The listing builds one solid part. Answer for the finished solid, in the listing's coordinates (mm). Face numbers are marked on the shaded views. A direction names the side the tool comes from. Coordinates: 2 decimals unless noted, no trailing zeros. Order: outer loops, then holes, each group sorted by start corner. A loop starts at its lowest first (then second) coordinate and runs counter-clockwise, first axis right, second up. Notation, with made-up numbers: (66, 42) -> (113, 42) arc R16 ccw to (113, 48) -> close; hole circle Ø4 at (-20, 89). An arc over 180 degrees is marked (long way). Answer in a Markdown table with one row per item.
```python
from build123d import *

# Parameters (mm, degrees)
SKETCH_2_R          = 1.25
CUT_EXTRUDE_1_DEPTH = 10
CUT_EXTRUDE_START   = -54.1
SKETCH_2_2_R        = 1.25
CUT_EXTRUDE_2_DEPTH = 6
SKETCH_3_OUTSIDE_W  = 33.054
SKETCH_3_OUTSIDE_H  = 33.054
SKETCH_3_OUTSIDE_R  = 8.75
CUT_EXTRUDE_3_DEPTH = 20.1
SKETCH_4_R          = 5.25
SKETCH_4_R_2        = 4.25
EXTRUDE_1_DEPTH     = 4


with BuildPart() as part:
    # 草图1 → 旋转1 (revolve)
    with BuildSketch(Plane.XY, mode=Mode.PRIVATE) as revolve_1_sk:
        Polygon((-9, 36), (-5.25, 36), (-5.25, 5), (-9, 5), (-9, 0), (-4.25, 0), (-4.25, 60.1), (-9, 60.1), align=None)
    revolve(revolve_1_sk.sketch.rotate(Axis((0, 0, 0), (0, 1, 0)), 270), axis=Axis((0, 0, 0), (0, 1, 0)))

    # 草图2 → 切除-拉伸1 (cut)
    with BuildSketch(Plane(origin=(0, 60.1, 0), x_dir=(1, 0, 0), z_dir=(0, 1, 0))):
        with Locations(Location((0, 7, 0), (0, 0, 270))):
            Circle(SKETCH_2_R)
        with Locations(Location((0, -7, 0), (0, 0, 270))):
            Circle(SKETCH_2_R)
        with Locations(Location((-7, 0, 0), (0, 0, 270))):
            Circle(SKETCH_2_R)
        with Locations(Location((7, 0, 0), (0, 0, 270))):
            Circle(SKETCH_2_R)
    extrude(amount=-CUT_EXTRUDE_1_DEPTH, mode=Mode.SUBTRACT)

    # 草图2<2> → 切除-拉伸2 (cut)
    with BuildSketch(Plane(origin=(0, 60.1, 0), x_dir=(1, 0, 0), z_dir=(0, 1, 0)).offset(CUT_EXTRUDE_START)):
        with Locations(Location((0, 7, 0), (0, 0, 270))):
            Circle(SKETCH_2_2_R)
        with Locations(Location((0, -7, 0), (0, 0, 270))):
            Circle(SKETCH_2_2_R)
        with Locations(Location((-7, 0, 0), (0, 0, 270))):
            Circle(SKETCH_2_2_R)
        with Locations(Location((7, 0, 0), (0, 0, 270))):
            Circle(SKETCH_2_2_R)
    extrude(amount=-CUT_EXTRUDE_2_DEPTH, mode=Mode.SUBTRACT)

    # 草图3 outside → 切除-拉伸3 (cut)
    with BuildSketch(Plane(origin=(0, 60.1, 0), x_dir=(1, 0, 0), z_dir=(0, 1, 0))):
        Rectangle(SKETCH_3_OUTSIDE_W, SKETCH_3_OUTSIDE_H)
        with Locations(Location((0, 0, 0), (0, 0, 270))):
            Circle(SKETCH_3_OUTSIDE_R, mode=Mode.SUBTRACT)
    extrude(amount=-CUT_EXTRUDE_3_DEPTH, mode=Mode.SUBTRACT)

    # 草图4 → 凸台-拉伸1 (add)
    with BuildSketch(Plane(origin=(0, 60.1, 0), x_dir=(1, 0, 0), z_dir=(0, 1, 0))):
        with Locations(Location((0, 0, 0), (0, 0, 90))):
            Circle(SKETCH_4_R)
        with Locations(Location((0, 0, 0), (0, 0, 90))):
            Circle(SKETCH_4_R_2, mode=Mode.SUBTRACT)
    extrude(amount=EXTRUDE_1_DEPTH)


solid = part.part
```
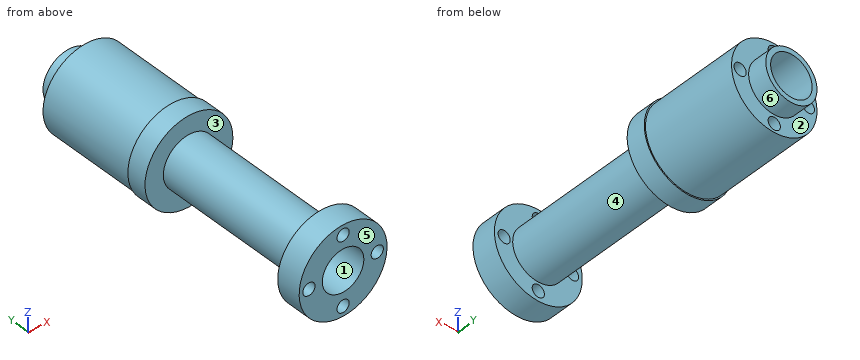
(1) A cutting plane is placed at A-A, the plane x = -2.25. Determine the outline of the cut face in (y, z).
Check values:
| item | result |
|---|---|
| outline | (0, -8.71) -> (5, -8.71) -> (5, -4.74) -> (36, -4.74) -> (36, -8.71) -> (40, -8.71) -> (40, -8.46) -> (60.1, -8.46) -> (60.1, -4.74) -> (64.1, -4.74) -> (64.1, -3.61) -> (0, -3.61) -> close; (0, 3.61) -> (64.1, 3.61) -> (64.1, 4.74) -> (60.1, 4.74) -> (60.1, 8.46) -> (40, 8.46) -> (40, 8.71) -> (36, 8.71) -> (36, 4.74) -> (5, 4.74) -> (5, 8.71) -> (0, 8.71) -> close |
(2) A cutting plane is placed at B-B, the plane z = -2.5. Determine the outline of the cut face in (x, y), then the cut area to 3 significant figures.
Check values:
| item | result |
|---|---|
| outline | (-8.65, 0) -> (-3.44, 0) -> (-3.44, 64.1) -> (-4.62, 64.1) -> (-4.62, 60.1) -> (-8.39, 60.1) -> (-8.39, 40) -> (-8.65, 40) -> (-8.65, 36) -> (-4.62, 36) -> (-4.62, 5) -> (-8.65, 5) -> close; (3.44, 0) -> (8.65, 0) -> (8.65, 5) -> (4.62, 5) -> (4.62, 36) -> (8.65, 36) -> (8.65, 40) -> (8.39, 40) -> (8.39, 60.1) -> (4.62, 60.1) -> (4.62, 64.1) -> (3.44, 64.1) -> close |
| area | 375 mm² |
(3) Flat-ended cylindrical pins translate along their axes: pin 1 (1.5 mm diameter, centred on x = 5, y = 37.5, fed in from -Z); pin 2 (1 mm diameter, centred on x = -3, y = 43, fed in from -Z); pin 3 (8 mm diameter, centred on y = 15, z = 6, fed in from +X). Find the tip coordinate at first contact, or state that the pin passes through.
Check values:
| item | result |
|---|---|
| pin 1 | z = -7.93 |
| pin 2 | z = -8.39 |
| pin 3 | x = 4.85 |
(4) A cutting plane is placed at C-C, the plane z = -7. Determine the outline of the cut face in (x, y).
Check values:
| item | result |
|---|---|
| outline | (-5.66, 0) -> (-1.25, 0) -> (-1.25, 5) -> (-5.66, 5) -> close; (-5.66, 36) -> (5.66, 36) -> (5.66, 40) -> (5.25, 40) -> (5.25, 60.1) -> (1.25, 60.1) -> (1.25, 50.1) -> (-1.25, 50.1) -> (-1.25, 60.1) -> (-5.25, 60.1) -> (-5.25, 40) -> (-5.66, 40) -> close; (1.25, 0) -> (5.66, 0) -> (5.66, 5) -> (1.25, 5) -> close |
(5) For a pull along Y with two mould halves and no side action, classify the marked faces 4, 5 and 6 as released by +Y, released by -Y, zero draft, split by the parting line, or undercut.
Check values:
| item | result |
|---|---|
| face 4 | undercut |
| face 5 | released by -Y |
| face 6 | zero draft |
(6) A cutting plane is placed at D-D, the plane y = 32. Determine the outline of the cut face in (x, z), then the cut area to 3 significant figures.
Check values:
| item | result |
|---|---|
| outline | circle Ø10.5 at (0, 0); hole circle Ø8.5 at (0, 0) |
| area | 29.8 mm² |
(7) Which of the six approach directions +Z, -Z, +X, -X, +Y, -Y give full straight-line access (tool end or side, diameter ignored) to the marked faces 1, 2 and 3?
Check values:
| item | result |
|---|---|
| face 1 | +Y, -Y |
| face 2 | +Y |
| face 3 | none |
(8) Find the intervals of material crossed by line 1 along X through (y, z) = (3.75, 0); line 2 along X through (y, z) = (56.5, 0); line 3 along Y through (x, z) = (4.75, 5), in increasing order. Write a range as from..to.
Check values:
| item | result |
|---|---|
| line 1 | -9..-8.25, -5.75..-4.25, 4.25..5.75, 8.25..9 |
| line 2 | -8.75..-8.25, -5.75..-4.25, 4.25..5.75, 8.25..8.75 |
| line 3 | 0..5, 36..60.1 |
